Work out the finished part from the listing and answer in its coordinate system (mm). A direction names the side the tool comes from. Round coordinates to 2 decimals unless told otherwise and drop trailing zeros. Loops run counter-clockwise (first coordinate to the right, second up) from the corner with the lowest first, then second, coordinate; pieces in that order, holes last. Notation, with made-up numbers: (-32.75, 42.25) - (-2.75, 42.25) arc R16 ccw to (-2.75, 72.25) - close; hole circle Ø1 at (75, -32.75). An arc over 180 degrees is marked (long way). Return JSON: item names as keys, results as strings.
from build123d import *

# Parameters (mm, degrees)
F2_R     = 7.9
F3_DEPTH = 2
F5_DEPTH = 2
F6_R     = 7.5
F7_DEPTH = 2
F8_DEPTH = 1


with BuildPart() as f1:
    # F0 (on Front) → F1 (revolve)
    with BuildSketch(Plane.XZ):
        Polygon((2.5, 2.6889840401), (2.5, -0.3110159599), (9.5, -0.3110159599), (9.5, 1.6889840401), (7.5, 2.6889840401), align=None)
    revolve(axis=Axis((0, 0, 1.1889840401), (0, 0, -1)))

    # F2 (on face) → F3 (join)
    with BuildSketch(Plane(origin=(0, 0, -0.3110159599), x_dir=(1, 0, 0), z_dir=(0, 0, -1))):
        Circle(F2_R)
    extrude(amount=F3_DEPTH)

    # F4 (on face) → F5 (cut)
    with BuildSketch(Plane(origin=(0, 0, -2.3110159599), x_dir=(1, 0, 0), z_dir=(0, 0, -1))):
        with BuildLine():
            ThreePointArc((2.1354156504, -1.3), (2.4071289045, -0.675078097), (2.5, 0))
            ThreePointArc((2.5, 0), (2.4071289045, 0.675078097), (2.1354156504, 1.3))
            Line((2.1354156504, 1.3), (-2.1354156504, 1.3))
            ThreePointArc((-2.1354156504, 1.3), (-2.5, 0), (-2.1354156504, -1.3))
            Line((-2.1354156504, -1.3), (2.1354156504, -1.3))
        make_face()
        with BuildLine():
            ThreePointArc((2.1354156504, 1.3), (2.4071289045, 0.675078097), (2.5, 0))
            ThreePointArc((2.5, 0), (2.4071289045, -0.675078097), (2.1354156504, -1.3))
            Line((2.1354156504, -1.3), (8.2728397101, -1.3))
            Line((8.2728397101, -1.3), (8.2728397101, 1.3))
            Line((8.2728397101, 1.3), (2.1354156504, 1.3))
        make_face()
        with BuildLine():
            Line((-2.1354156504, 1.3), (2.1354156504, 1.3))
            ThreePointArc((2.1354156504, 1.3), (0, 2.5), (-2.1354156504, 1.3))
        make_face()
        with BuildLine():
            ThreePointArc((-2.1354156504, -1.3), (0, -2.5), (2.1354156504, -1.3))
            Line((2.1354156504, -1.3), (-2.1354156504, -1.3))
        make_face()
        with BuildLine():
            ThreePointArc((-2.1354156504, -1.3), (-2.5, 0), (-2.1354156504, 1.3))
            Line((-2.1354156504, 1.3), (-8.2728397101, 1.3))
            Line((-8.2728397101, 1.3), (-8.2728397101, -1.3))
            Line((-8.2728397101, -1.3), (-2.1354156504, -1.3))
        make_face()
    extrude(amount=-F5_DEPTH, mode=Mode.SUBTRACT)

    # F6 (on face) → F7 (cut)
    with BuildSketch(Plane.XY.offset(2.6889840401)):
        Circle(F6_R)
    extrude(amount=-F7_DEPTH, mode=Mode.SUBTRACT)

    # F6 (on face) → F8 (cut)
    with BuildSketch(Plane.XY.offset(2.6889840401)):
        Circle(F6_R)
    extrude(amount=-F8_DEPTH, mode=Mode.SUBTRACT)


solid = f1.part
1) Determine the mould class of faces 4 (the cylindrical face through (0.16, -7.9, -1.3)), 5 (the flat face through (-2, 2, 0.689)), 6 (the flat face through (0, -4, -2.311)) for opening direction X: pulls with the +X half, pulls with the -X half, needs draft (parallel to the pull), parting line crosses it, or undercut.
Verdict:
{"face 4": "parting line crosses it", "face 5": "undercut", "face 6": "needs draft"}
2) Flat-ended cylindrical pins translate along their axes: pin 1 (2 mm diameter, centred on y = 7, z = 1.5, fed in from +X); pin 2 (6 mm diameter, centred on x = -1, y = -1.5, fed in from -Z); pin 3 (1 mm diameter, centred on x = -3.5, z = -1.5, fed in from +Y); pin 4 (1 mm diameter, centred on x = 5.5, z = -1.5, fed in from -Y). Find the tip coordinate at first contact, or state that the pin passes through.
Verdict:
{"pin 1": "stops at x = 7.37", "pin 2": "stops at z = -2.31", "pin 3": "stops at y = 7.31", "pin 4": "stops at y = -6.12"}
3) Section D-D (z = 0.4) is taken. Give the vertices of the cut face in (x, y).
Verdict:
{"outline": "circle Ø19 at (0, 0); hole circle Ø5 at (0, 0)"}
4) A tool of negligible diameter and unlimited length cuts with its end or side. For faces 1 (the cylindrical face through (-0.16, 7.9, -1.3)), 2 (the cylindrical face through (-7.493, 0.33, 1.703)), 3 (the flat face through (5, -1.3, -1)), from which of +Z, -Z, +X, -X, +Y, -Y can it reach the whole face along a straight path? Write none if from no direction.
Verdict:
{"face 1": "-Z, +Y", "face 2": "+Z", "face 3": "-Z, +X, -X"}
5) Find the intervals of material crossed by L1, parallel to X at y = 0.25, z = 1.3; L2, parallel to X at y = 0, z = -0.05, in increasing order.
Verdict:
{"L1": "x = -9.5 to -7.5, 7.5 to 9.5", "L2": "x = -9.5 to -2.5, 2.5 to 9.5"}
6) Section C-C (z = -0.8) is taken. Give the vertices of the cut face in (x, y), and give its area (3 significant figures).
Verdict:
{"outline": "(-7.79, -1.3) arc R7.9 ccw to (7.79, -1.3) - (2.14, -1.3) arc R2.5 cw to (-2.14, -1.3) - close; (-7.79, 1.3) - (-2.14, 1.3) arc R2.5 cw to (2.14, 1.3) - (7.79, 1.3) arc R7.9 ccw to start", "area": "148 mm2"}
7) Section B-B (y = 0) is taken. Give the vertices of the cut face in (x, z).
Verdict:
{"outline": "(-9.5, -0.31) - (-2.5, -0.31) - (-2.5, 0.69) - (-7.5, 0.69) - (-7.5, 2.69) - (-9.5, 1.69) - close; (2.5, -0.31) - (9.5, -0.31) - (9.5, 1.69) - (7.5, 2.69) - (7.5, 0.69) - (2.5, 0.69) - close"}
8) Section A-A (x = 0) is taken. Give the vertices of the cut face in (y, z).
Verdict:
{"outline": "(-9.5, -0.31) - (-7.9, -0.31) - (-7.9, -2.31) - (-2.5, -2.31) - (-2.5, 0.69) - (-7.5, 0.69) - (-7.5, 2.69) - (-9.5, 1.69) - close; (2.5, -2.31) - (7.9, -2.31) - (7.9, -0.31) - (9.5, -0.31) - (9.5, 1.69) - (7.5, 2.69) - (7.5, 0.69) - (2.5, 0.69) - close"}
